Part model, mm, in its own coordinate system. Face numbers are marked on the shaded views. A direction names the side the tool comes from. Round coordinates to 2 decimals unless told otherwise and drop trailing zeros. Loops run counter-clockwise (first coordinate to the right, second up) from the corner with the lowest first, then second, coordinate; pieces in that order, holes last. Notation, with made-up numbers: (13.25, 24.25) -> (17.25, 24.25) arc R20 ccw to (17.25, 30.25) -> close; hole circle Ø6 at (17.25, 13). An arc over 180 degrees is marked (long way). Use a Markdown table: item, result. Add a question column.
Item 1: Flat gauge pins, fed straight in: pin 1 (2.5 mm diameter, centred on x = 6, z = -10.5, fed in from -Y); pin 2 (1.5 mm diameter, centred on x = 35.5, y = 12, fed in from -Z); pin 3 (11.5 mm diameter, centred on y = 18, z = -24.5, fed in from -X); pin 4 (1.5 mm diameter, centred on x = 54, z = -44, fed in from -Y). Where does each tip first touch, or does it go through?
Item 2: Which spindle directions (+Z, -Z, +X, -X, +Y, -Y) get a long thin tool onto all of the face, cutting with end or side? Do the marked faces 4, 5, 6, 7 and 8. Say none if no direction does.
Item 3: Cut at C-C, the plane x = 53.34. List the corners of the cut face in (y, z) (3 decimals), plus the area to 3 significant figures.
Item 4: Cut at B-B, the plane y = 1. List the corners of the cut face in (x, z), plus the area to 3 significant figures.
Item 5: Cut at A-A, the plane z = -10.16. List the corners of the cut face in (x, y) (3 decimals), plus the area to 3 significant figures.
Item 6: Probe line 1 (X direction, y = -1, z = -10); line 2 (Z direction, x = 5.08, y = -0.1) (3 decimals); line 3 (Y direction, x = 53.5, z = -29). List the from-to ranges inside material, lowest first. Write a range as [from, to].
Item 7: Two-plate mould, pull along Y, no slides. Class the marked faces 1, 2 and 3: pulls with the +Y half, pulls with the -Y half, needs draft (parallel to the pull), parting line crosses it, or undercut.
Item 8: Cut at D-D, the plane x = 20.5. List the corners of the cut face in (y, z).
```python
from build123d import *

# Parameters (mm, degrees)
SKETCH1_R           = 2
BOSS_EXTRUDE1_DEPTH = 2
SKETCH2_W           = 43
SKETCH2_H           = 25
BOSS_EXTRUDE2_DEPTH = 23
SKETCH4_R           = 5
BOSS_EXTRUDE3_DEPTH = 14.39
SKETCH5_R           = 2.555
SKETCH5_R_2         = 2
BOSS_EXTRUDE4_DEPTH = 4
SKETCH6_W           = 25
SKETCH6_H           = 10
BOSS_EXTRUDE5_DEPTH = 20


with BuildPart() as part:
    # Sketch1 → Boss-Extrude1 (new body)
    with BuildSketch(Plane(origin=(0, 0, 0), x_dir=(1, 0, 0), z_dir=(0, 1, 0))):
        Polygon((55.88, 48.26), (63.507713889, 35.565352277), (73.667713889, 35.565352277), (73.667713889, 22.865352277), (66.047713889, 22.865352277), (58.42, 12.7), (58.42, 0), (0, 0), (0, 17.78), (5.08, 17.78), (5.08, 48.26), align=None)
        with Locations((5.08, 10.16)):
            Circle(SKETCH1_R, mode=Mode.SUBTRACT)
        with Locations((53.34, 10.16)):
            Circle(SKETCH1_R, mode=Mode.SUBTRACT)
        with Locations((53.34, 43.18)):
            Circle(SKETCH1_R, mode=Mode.SUBTRACT)
    extrude(amount=BOSS_EXTRUDE1_DEPTH)

    # Sketch2 → Boss-Extrude2 (add)
    with BuildSketch(Plane(origin=(0, 2, 0), x_dir=(1, 0, 0), z_dir=(0, 1, 0))):
        with Locations((28.58, 30.5)):
            Rectangle(SKETCH2_W, SKETCH2_H)
    extrude(amount=BOSS_EXTRUDE2_DEPTH)

    # Sketch4 → Boss-Extrude3 (add)
    with BuildSketch(Plane.XZ):
        with Locations((68.587713889, -29.215352277)):
            Circle(SKETCH4_R)
    extrude(amount=BOSS_EXTRUDE3_DEPTH)

    # Sketch5 → Boss-Extrude4 (add)
    with BuildSketch(Plane.XZ):
        with Locations((5.08, -10.16)):
            Circle(SKETCH5_R)
        with Locations((5.08, -10.16)):
            Circle(SKETCH5_R_2, mode=Mode.SUBTRACT)
        with Locations((53.34, -10.16)):
            Circle(SKETCH5_R)
        with Locations((53.34, -10.16)):
            Circle(SKETCH5_R_2, mode=Mode.SUBTRACT)
        with Locations((53.34, -43.18)):
            Circle(SKETCH5_R)
        with Locations((53.34, -43.18)):
            Circle(SKETCH5_R_2, mode=Mode.SUBTRACT)
    extrude(amount=BOSS_EXTRUDE4_DEPTH)

    # Sketch6 → Boss-Extrude5 (add)
    with BuildSketch(Plane(origin=(0, 0, -43), x_dir=(-1, 0, 0), z_dir=(0, 0, -1))):
        with Locations((-28.58, 20)):
            Rectangle(SKETCH6_W, SKETCH6_H)
    extrude(amount=BOSS_EXTRUDE5_DEPTH)


solid = part.part
```
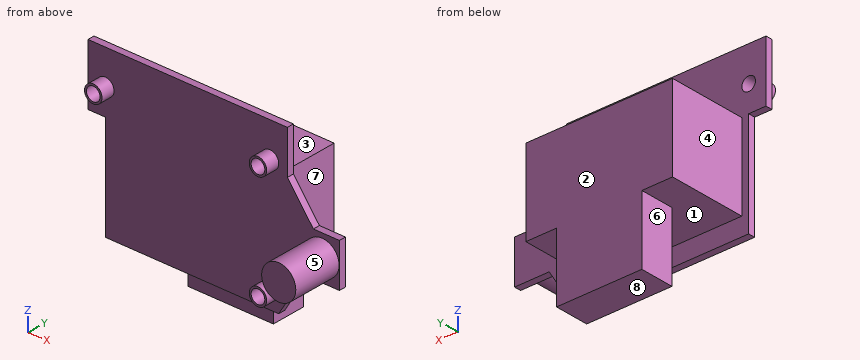
A:
| question | item | result |
|---|---|---|
| 1 | pin 1 | stops at y = -4 |
| 1 | pin 2 | stops at z = -43 |
| 1 | pin 3 | stops at x = 7.08 |
| 1 | pin 4 | passes through |
| 2 | face 4 | +Z, -Z, -X, +Y |
| 2 | face 5 | -Y |
| 2 | face 6 | -Z, -X, +Y |
| 2 | face 7 | +Z, -Z, +X, +Y |
| 2 | face 8 | -Z, +X, -X, +Y, -Y |
| 3 | outline | (-4, -45.735) -> (0, -45.735) -> (0, -48.26) -> (2, -48.26) -> (2, -45.18) -> (-4, -45.18) -> close; (-4, -41.18) -> (2, -41.18) -> (2, -12.16) -> (-4, -12.16) -> (-4, -12.715) -> (0, -12.715) -> (0, -40.625) -> (-4, -40.625) -> close; (-4, -8.16) -> (2, -8.16) -> (2, 0) -> (0, 0) -> (0, -7.605) -> (-4, -7.605) -> close |
| 3 | area | 89.4 mm^2 |
| 4 | outline | (0, -17.78) -> (5.08, -17.78) -> (5.08, -48.26) -> (55.88, -48.26) -> (63.51, -35.57) -> (73.67, -35.57) -> (73.67, -22.87) -> (66.05, -22.87) -> (58.42, -12.7) -> (58.42, 0) -> (0, 0) -> close; hole circle Ø4 at (5.08, -10.16); hole circle Ø4 at (53.34, -43.18); hole circle Ø4 at (53.34, -10.16) |
| 4 | area | 2,880 mm^2 |
| 5 | outline | (0, 0) -> (2.525, 0) -> (2.525, -4) -> (3.08, -4) -> (3.08, 2) -> (0, 2) -> close; (7.08, -4) -> (7.635, -4) -> (7.635, 0) -> (50.785, 0) -> (50.785, -4) -> (51.34, -4) -> (51.34, 2) -> (7.08, 2) -> close; (55.34, -4) -> (55.895, -4) -> (55.895, 0) -> (58.42, 0) -> (58.42, 2) -> (55.34, 2) -> close |
| 5 | area | 110 mm^2 |
| 6 | line 1 | x = [2.53, 3.09], [7.07, 7.63], [50.79, 51.35], [55.33, 55.89] |
| 6 | line 2 | z = [-12.715, -12.16], [-8.16, -7.605] |
| 6 | line 3 | y = [0, 2] |
| 7 | face 1 | undercut |
| 7 | face 2 | pulls with the +Y half |
| 7 | face 3 | needs draft |
| 8 | outline | (0, -48.26) -> (2, -48.26) -> (2, -43) -> (15, -43) -> (15, -63) -> (25, -63) -> (25, -18) -> (2, -18) -> (2, 0) -> (0, 0) -> close |
